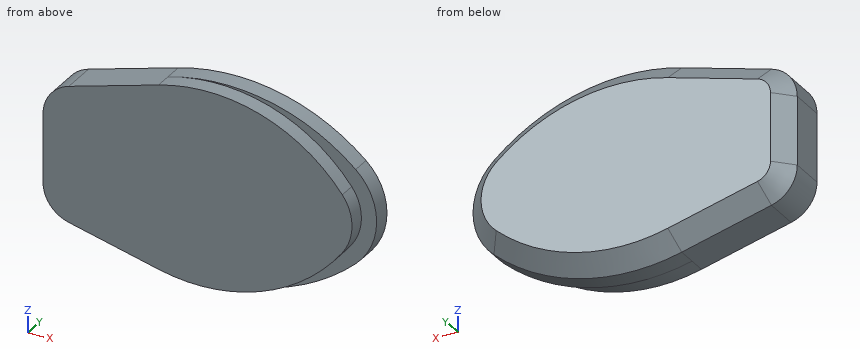
Autodesk Inventor part; units mm, degrees
ref_plane "YZ Plane" through (0, 0, 0) normal (1, 0, 0) x (0, 1, 0)
ref_plane "XZ Plane" through (0, 0, 0) normal (0, 1, 0) x (-1, 0, 0)
ref_plane "XY Plane" through (0, 0, 0) normal (0, 0, 1) x (1, 0, 0)
sketch "Sketch1" plane through (0, 0, 0) normal (0, 1, 0) x (-1, 0, 0)
  circle A0 centre (0, 0) radius 5.5
  line L0 (0, 0) -> (30, 0) construction
  line L1 (30, -7) -> (30, 7)
  line L2 (30, -7) -> (16.7292, -10.5559)
  arc A1 (-4.3821, -3.3237) -> (16.7292, -10.5559) centre (11.5528, 8.7626) ccw
  line L3 (30, 7) -> (16.7292, 10.5559)
  arc A2 (16.7292, 10.5559) -> (-4.3821, 3.3237) centre (11.5528, -8.7626) ccw
  circle A3 centre (0, 0) radius 7.25
  arc A4 (16.7292, 10.5559) -> (-4.8424, 5.3957) centre (10.7046, -11.928) ccw
  arc A5 (-4.8424, -5.3957) -> (16.7292, -10.5559) centre (10.7046, 11.928) ccw
  point P0 (1.7838, 5.2027)
  point P1 (1.7838, -5.2027)
  point P2 (16.7292, 10.5559)
  point P3 (30, 9.4853)
  point P4 (30, -9.4853)
  point P5 (30, -9.4752)
  point P6 (30, 9.4752)
  dimension "d0" = 11
  dimension "d1" = 30
  dimension "d2" = 14
  dimension "d5" = 30
  dimension "d10" = 14.5
  dimension "d52" = 20
extrude "Extrusion1" add sketch "Sketch1" against normal blind 2 contours A0 | A0 A2 A3 A1 | A2 L3 L1 L2 A1 A3 picked at (6.6012, -0.5586)
extrude "Extrusion2" add sketch "Sketch1" along normal blind 4.2
fillet "Fillet1" radius 4 2 edges at (-30, 1.1, 7) (-30, 1.1, -7)
chamfer "Chamfer1" distance 2 angle 45 8 edges at (-30, 4.2, 0) (-29.1734, 4.2, 6.3657) (-21.8822, 4.2, 9.1752) (-5.2893, 4.2, 10.7104) (7.25, 4.2, 0) (-5.2893, 4.2, -10.7104) (-21.8822, 4.2, -9.1752) (-29.1734, 4.2, -6.3657)
sketch "Sketch9" plane through (0, -2, 0) normal (0, -1, 0) x (1, 0, 0)
  arc A0 (-27.0353, 7.7944) -> (-30, 3.9307) centre (-26, 3.9307) ccw
  line L0 (-30, 3.9307) -> (-30, -3.9307)
  arc A1 (-30, -3.9307) -> (-27.0353, -7.7944) centre (-26, -3.9307) ccw
  arc A2 (6.1782, -6.8842) -> (6.1782, 6.8842) centre (0, 0) ccw
  line L1 (-32, -3.9307) -> (-32, 3.9307)
  line L2 (-27.5363, -9.7307) -> (-33.6527, -8.0918)
  arc A3 (-36.9536, -3.79) -> (-33.6527, -8.0918) centre (-32.5, -3.79) ccw
  line L3 (-36.9536, -3.79) -> (-36.9536, 4.2596)
  arc A4 (-33.0372, 8.6806) -> (-36.9536, 4.2596) centre (-32.5, 4.2596) ccw
  line L4 (-32, 3.9307) -> (-32, -3.9307)
  line L5 (-26.7661, 9.4426) -> (-33.0372, 8.6806)
  arc A5 (-17.2468, -12.4878) -> (6.1782, -6.8842) centre (-10.7046, 11.928) ccw
  line L6 (-26.5589, -7.4525) -> (-33.0176, -5.7218)
  arc A6 (-34.5, -3.79) -> (-33.0176, -5.7218) centre (-32.5, -3.79) ccw
  line L7 (-34.5, -3.79) -> (-34.5, 4.2596)
  arc A7 (-33.0176, 6.1914) -> (-34.5, 4.2596) centre (-32.5, 4.2596) ccw
  line L8 (-33.0176, 6.1914) -> (-27.0353, 7.7944)
  arc A8 (4.3821, 3.3237) -> (-16.7292, 10.5559) centre (-11.5528, -8.7626) ccw
  arc A9 (-16.7292, -10.5559) -> (4.3821, -3.3237) centre (-11.5528, 8.7626) ccw
  arc A10 (4.3821, -3.3237) -> (4.3821, 3.3237) centre (0, 0) ccw
  arc A11 (4.3821, 3.3237) -> (-16.7292, 10.5559) centre (-11.5528, -8.7626) ccw
  line L9 (-16.7292, 10.5559) -> (-27.0353, 7.7944)
  line L10 (-27.0353, -7.7944) -> (-16.7292, -10.5559)
  arc A12 (-17.2468, -12.4878) -> (6.1782, -6.8842) centre (-10.7046, 11.928) ccw
  line L11 (-17.2468, -12.4878) -> (-27.5529, -9.7262)
  arc A13 (-32, -3.9307) -> (-27.5529, -9.7262) centre (-26, -3.9307) ccw
  arc A14 (-27.5529, 9.7262) -> (-32, 3.9307) centre (-26, 3.9307) ccw
  line L12 (-27.5529, 9.7262) -> (-17.2468, 12.4878)
  arc A15 (6.1782, 6.8842) -> (-17.2468, 12.4878) centre (-10.7046, -11.928) ccw
  line L13 (-27.5529, -9.7262) -> (-17.2468, -12.4878)
  line L14 (-27.0353, 7.7944) -> (-16.7292, 10.5559)
  point P0 (-27.5529, -9.7262)
  point P1 (-31.5927, -6.1037)
  point P2 (-31.355, 6.6369)
  point P3 (-28.9, 9.1833)
  dimension "d90" = 2.5
  dimension "d91" = 2
sketch "Sketch11" plane through (0, 6.1, 0) normal (0, 1, 0) x (1, 0, 0)
  arc A0 (4.0599, -4.5238) -> (4.0599, 4.5238) centre (0, 0) ccw
  line L0 (-28.8284, -3.9307) -> (-28.8284, 3.9307)
  line L1 (-26.7321, 6.6627) -> (-16.4259, 9.4243)
  arc A1 (4.0599, 4.5238) -> (-16.4259, 9.4243) centre (-10.7046, -11.928) ccw
  arc A2 (-16.4259, -9.4243) -> (4.0599, -4.5238) centre (-10.7046, 11.928) ccw
  line L2 (-16.4259, -9.4243) -> (-26.7321, -6.6627)
  arc A3 (-28.8284, -3.9307) -> (-26.7321, -6.6627) centre (-26, -3.9307) ccw
  arc A4 (-26.7321, 6.6627) -> (-28.8284, 3.9307) centre (-26, 3.9307) ccw
  dimension "d75" = 1
  dimension "d76" = 1
  dimension "d77" = 1
  dimension "d78" = 10
  dimension "d79" = 80
sketch "Sketch16" plane through (0, 11.1, 0) normal (0, 1, 0) x (1, 0, 0)
  point P0 (0, 0)
sketch "Sketch15" plane through (-28, 4.1, -3.9307) normal (0, -1, 0) x (1, 0, 0)
  point P0 (28, 3.9307)
  point P1 (28, 3.9307)
properties part number "FS-00-SLBV8"
Could you check a few things on this model? Use its own coordinates, in mm. Coordinates: 2 decimals unless noted, no trailing zeros. Order: outer loops, then holes, each group sorted by start corner. A loop starts at its lowest first (then second) coordinate and runs counter-clockwise, first axis right, second up. Notation, with made-up numbers: M 67,47 L 117,47 A19 cw 117,60 Z; hole C 63.25,-16 d6. An arc over 180 degrees is marked long. Use a Markdown table: item, result. Add a question column.
Q1. I want a section at A-A on y = 3. List the corners of the cut face in (x, z) for me, then the cut area to 3 significant figures.
Q2. If I drill on L1, parallel to X at y = -0.75, z = -0.25; L2, parallel to Z at x = -11, y = 0.75; L3, parallel to X at y = 2, z = 1.75, over which ranges is the centre line in solid material (lowest first)?
Q3. I'm going to push a flat-ended pin straight in: pin 1 (2 mm diameter, centred on y = -0.5, z = 8, fed in from -X) (3 decimals). Where does the tip first touch, or does it pass through?
Q4. I want a section at B-B on x = -21.5. List the corners of the cut face in (y, z) for me.
Q5. I want a section at C-C on y = -0.75. List the corners of the cut face in (x, z) for me, then the cut area to 3 significant figures.
Checked values:
| question | item | result |
|---|---|---|
| 1 | outline | M -29.2,-3.93 A3.2 ccw -26.83,-7.02 L -16.52,-9.78 A22.48 ccw 4.31,-4.8 A6.45 ccw 4.31,4.8 A22.48 ccw -16.52,9.78 L -26.83,7.02 A3.2 ccw -29.2,3.93 Z |
| 1 | area | 599 mm² |
| 2 | L1 | -30 to 5.49 |
| 2 | L2 | -11.35 to 11.35 |
| 2 | L3 | -30 to 7.04 |
| 3 | pin 1 | x = -28.565 |
| 4 | outline | M -2,-9.28 L 2.2,-9.28 L 4.2,-7.21 L 4.2,7.21 L 2.2,9.28 L -2,9.28 Z |
| 5 | outline | M -30,-3.93 A4 ccw -27.04,-7.79 L -16.73,-10.56 A20 ccw 4.38,-3.32 A5.5 ccw 4.38,3.32 A20 ccw -16.73,10.56 L -27.04,7.79 A4 ccw -30,3.93 Z |
| 5 | area | 631 mm² |
